Geometry: see drawing. Coordinates: mm, zero at the bounding-box minimum. A direction names the side the tool comes from. Round coordinates to 2 decimals unless told otherwise and drop trailing zeros. Write each loop counter-clockwise with the first axis right and the second up, starting at its lowest first coordinate (ties: lowest second). Pieces come first, ordered by that corner, then holes.
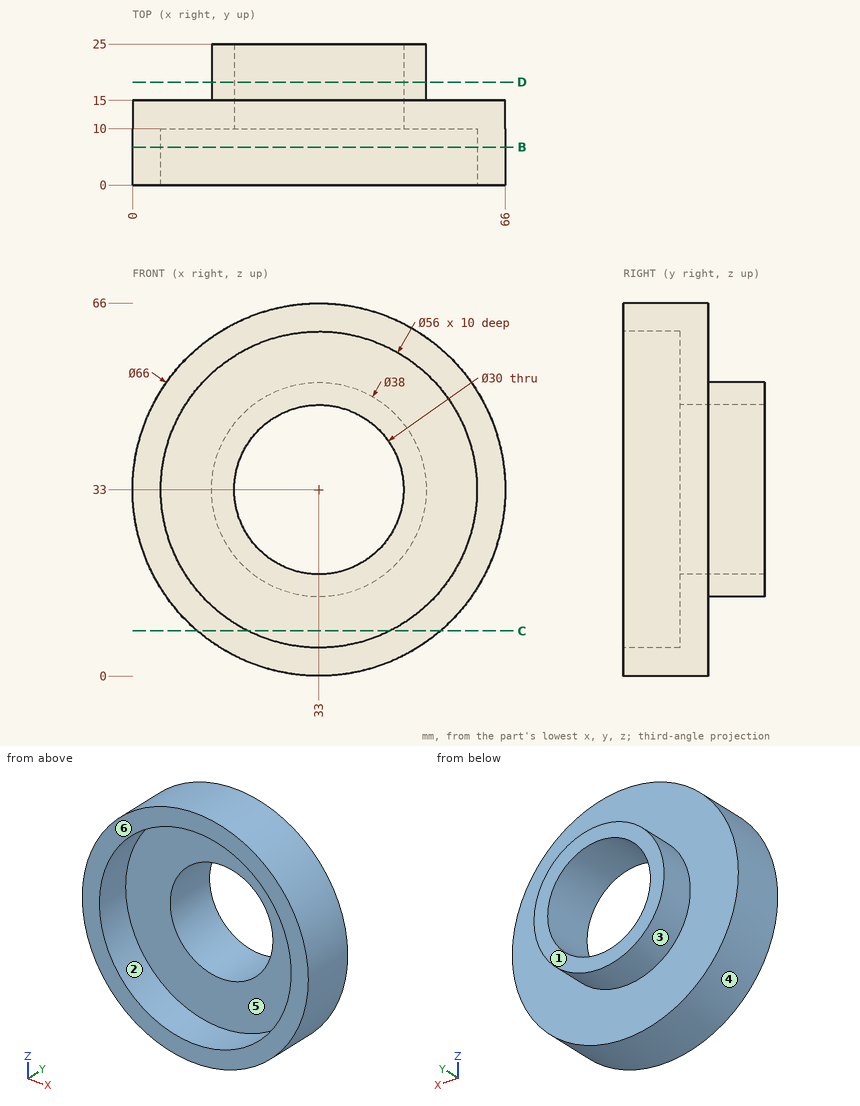
1) Pull-direction query (X, two-part tool) for the marked faces 4, 5 and 6; classes: released by +X, released by -X, zero draft, split by the parting line, or undercut.
Taken from the geometry:
face 4: split by the parting line
face 5: undercut
face 6: zero draft
2) Section query C-C on z = 8. Return the cut outline in (x, y).
Taken from the geometry:
outline: (11.46, 0) - (20.39, 0) - (20.39, 10) - (45.61, 10) - (45.61, 0) - (54.54, 0) - (54.54, 15) - (11.46, 15) - close
3) Reachability of the marked faces 1, 2 and 3 from +Z, -Z, +X, -X, +Y, -Y: full face, straight path, thin tool, end or side. Return the list, or none.
Taken from the geometry:
face 1: +Z, -Z, +X, -X, +Y
face 2: -Y
face 3: +Y
4) Section query B-B on y = 6.75. Return the cut outline in (x, z), then the cut area to 3 significant figures.
Taken from the geometry:
outline: circle Ø66 at (33, 33); hole circle Ø56 at (33, 33)
area: 958 mm2
5) Section query D-D on y = 18.25. Return the cut outline in (x, z), then the cut area to 3 significant figures.
Taken from the geometry:
outline: circle Ø38 at (33, 33); hole circle Ø30 at (33, 33)
area: 427 mm2
6) Material intervals for line 1 (Z direction, x = 33, y = 14); line 2 (X direction, y = 20.75, z = 33), sorted ascending.
Taken from the geometry:
line 1: z = 0 to 18, 48 to 66
line 2: x = 14 to 18, 48 to 52
7) Contact query for flat-ended pins moving along their axis: P1, Ø10, axis at y = 18.5, z = 29, coming from the +X side; P2, Ø8, axis at x = 46, y = 13, coming from the +Z side; P3, Ø6, axis at y = 6, z = 57.5, coming from the +X side (3 decimals). Output: stop coordinate, or through.
Taken from the geometry:
P1: stops at x = 66
P2: stops at z = 64.75
P3: stops at x = 58.035
